For this review, take the finished solid that the model builds, in its own axes (mm). A direction names the side the tool comes from. Coordinates: 2 decimals unless noted, no trailing zeros. Loops run counter-clockwise (first coordinate to the right, second up) from the corner with the lowest first, then second, coordinate; pieces in that order, holes last. Notation, with made-up numbers: (69.5, -15.5) -> (127.5, -15.5) arc R17 cw to (127.5, -8.5) -> close; hole circle Ø8 at (-0.75, 14). An arc over 180 degrees is marked (long way). One line per item, written item: value.
from build123d import *

# Parameters (mm, degrees)
F1_DEPTH = 40
F2_W     = 65
F2_H     = 40
F3_DEPTH = 5
F5_DEPTH = 6


with BuildPart() as f1:
    # F0 (on Top) → F1 (new body)
    with BuildSketch(Plane.XY):
        with BuildLine():
            Line((-3, 43), (1.2426406871, 43))
            ThreePointArc((1.2426406871, 43), (-6, 46), (-3, 38.7573593129))
            Line((-3, 38.7573593129), (-3, 43))
        make_face()
        with BuildLine():
            ThreePointArc((-3, 38.7573593129), (-1.3764116996, 39.0803111054), (0, 40))
            ThreePointArc((0, 40), (0.9196888946, 41.3764116996), (1.2426406871, 43))
            Line((1.2426406871, 43), (-3, 43))
            Line((-3, 43), (-3, 38.7573593129))
        make_face()
        with BuildLine():
            ThreePointArc((-3, 1.2426406871), (-1.3764116996, 0.9196888946), (0, 0))
            Line((0, 0), (0, 40))
            ThreePointArc((0, 40), (-1.3764116996, 39.0803111054), (-3, 38.7573593129))
            Line((-3, 38.7573593129), (-3, 1.2426406871))
        make_face()
        with BuildLine():
            ThreePointArc((1.2426406871, 43), (0.9196888946, 41.3764116996), (0, 40))
            Line((0, 40), (65, 40))
            ThreePointArc((65, 40), (64.0803111054, 41.3764116996), (63.7573593129, 43))
            Line((63.7573593129, 43), (1.2426406871, 43))
        make_face()
        with BuildLine():
            ThreePointArc((72.2426406871, 43), (68, 47.2426406871), (63.7573593129, 43))
            Line((63.7573593129, 43), (68, 43))
            Line((68, 43), (68, 38.7573593129))
            ThreePointArc((68, 38.7573593129), (71, 40), (72.2426406871, 43))
        make_face()
        with BuildLine():
            ThreePointArc((63.7573593129, 43), (64.0803111054, 41.3764116996), (65, 40))
            ThreePointArc((65, 40), (66.3764116996, 39.0803111054), (68, 38.7573593129))
            Line((68, 38.7573593129), (68, 43))
            Line((68, 43), (63.7573593129, 43))
        make_face()
        with BuildLine():
            ThreePointArc((72.2426406871, -3), (71, 0), (68, 1.2426406871))
            Line((68, 1.2426406871), (68, -3))
            Line((68, -3), (63.7573593129, -3))
            ThreePointArc((63.7573593129, -3), (68, -7.2426406871), (72.2426406871, -3))
        make_face()
        with BuildLine():
            ThreePointArc((68, 1.2426406871), (66.3764116996, 0.9196888946), (65, 0))
            ThreePointArc((65, 0), (64.0803111054, -1.3764116996), (63.7573593129, -3))
            Line((63.7573593129, -3), (68, -3))
            Line((68, -3), (68, 1.2426406871))
        make_face()
        with BuildLine():
            ThreePointArc((-3, 1.2426406871), (-6, -6), (1.2426406871, -3))
            Line((1.2426406871, -3), (-3, -3))
            Line((-3, -3), (-3, 1.2426406871))
        make_face()
        with BuildLine():
            ThreePointArc((1.2426406871, -3), (0.9196888946, -1.3764116996), (0, 0))
            ThreePointArc((0, 0), (-1.3764116996, 0.9196888946), (-3, 1.2426406871))
            Line((-3, 1.2426406871), (-3, -3))
            Line((-3, -3), (1.2426406871, -3))
        make_face()
        with BuildLine():
            Line((65, 0), (0, 0))
            ThreePointArc((0, 0), (0.9196888946, -1.3764116996), (1.2426406871, -3))
            Line((1.2426406871, -3), (63.7573593129, -3))
            ThreePointArc((63.7573593129, -3), (64.0803111054, -1.3764116996), (65, 0))
        make_face()
        with BuildLine():
            Line((65, 40), (65, 0))
            ThreePointArc((65, 0), (66.3764116996, 0.9196888946), (68, 1.2426406871))
            Line((68, 1.2426406871), (68, 38.7573593129))
            ThreePointArc((68, 38.7573593129), (66.3764116996, 39.0803111054), (65, 40))
        make_face()
    extrude(amount=F1_DEPTH)

    # F2 (on face) → F3 (join)
    with BuildSketch(Plane(origin=(0, 0, 0), x_dir=(1, 0, 0), z_dir=(0, 0, -1))):
        with BuildLine():
            Line((-3, -1.2426406871), (-3, -38.7573593129))
            ThreePointArc((-3, -38.7573593129), (-6, -46), (1.2426406871, -43))
            Line((1.2426406871, -43), (63.7573593129, -43))
            ThreePointArc((63.7573593129, -43), (71, -46), (68, -38.7573593129))
            Line((68, -38.7573593129), (68, -1.2426406871))
            ThreePointArc((68, -1.2426406871), (71, 6), (63.7573593129, 3))
            Line((63.7573593129, 3), (1.2426406871, 3))
            ThreePointArc((1.2426406871, 3), (-6, 6), (-3, -1.2426406871))
        make_face()
        with Locations((32.5, -20)):
            Rectangle(F2_W, F2_H, mode=Mode.SUBTRACT)
        with Locations((32.5, -20)):
            Rectangle(F2_W, F2_H)
    extrude(amount=F3_DEPTH)

    # F4 (on face) → F5 (join)
    with BuildSketch(Plane.XY):
        with BuildLine():
            ThreePointArc((22, 35), (16.8786796564, 37.1213203436), (19, 32))
            Line((19, 32), (19, 33.65))
            ThreePointArc((19, 33.65), (18.0454058454, 35.9545941546), (20.35, 35))
            Line((20.35, 35), (22, 35))
        make_face()
        with BuildLine():
            Line((19, 33.65), (19, 32))
            ThreePointArc((19, 32), (21.1213203436, 32.8786796564), (22, 35))
            Line((22, 35), (20.35, 35))
            ThreePointArc((20.35, 35), (19.9545941546, 34.0454058454), (19, 33.65))
        make_face()
        with BuildLine():
            Line((46, 33.65), (46, 32))
            ThreePointArc((46, 32), (48.1213203436, 32.8786796564), (49, 35))
            ThreePointArc((49, 35), (46, 38), (43, 35))
            Line((43, 35), (44.65, 35))
            ThreePointArc((44.65, 35), (46, 36.35), (47.35, 35))
            ThreePointArc((47.35, 35), (46.9545941546, 34.0454058454), (46, 33.65))
        make_face()
        with BuildLine():
            ThreePointArc((43, 35), (43.8786796564, 32.8786796564), (46, 32))
            Line((46, 32), (46, 33.65))
            ThreePointArc((46, 33.65), (45.0454058454, 34.0454058454), (44.65, 35))
            Line((44.65, 35), (43, 35))
        make_face()
        with BuildLine():
            ThreePointArc((19, 6.35), (19.9545941546, 5.9545941546), (20.35, 5))
            Line((20.35, 5), (22, 5))
            ThreePointArc((22, 5), (21.1213203436, 7.1213203436), (19, 8))
            Line((19, 8), (19, 6.35))
        make_face()
        with BuildLine():
            Line((22, 5), (20.35, 5))
            ThreePointArc((20.35, 5), (18.0454058454, 4.0454058454), (19, 6.35))
            Line((19, 6.35), (19, 8))
            ThreePointArc((19, 8), (16.8786796564, 2.8786796564), (22, 5))
        make_face()
        with BuildLine():
            ThreePointArc((46, 8), (43.8786796564, 7.1213203436), (43, 5))
            Line((43, 5), (44.65, 5))
            ThreePointArc((44.65, 5), (45.0454058454, 5.9545941546), (46, 6.35))
            Line((46, 6.35), (46, 8))
        make_face()
        with BuildLine():
            Line((44.65, 5), (43, 5))
            ThreePointArc((43, 5), (46, 2), (49, 5))
            ThreePointArc((49, 5), (48.1213203436, 7.1213203436), (46, 8))
            Line((46, 8), (46, 6.35))
            ThreePointArc((46, 6.35), (46.9545941546, 5.9545941546), (47.35, 5))
            ThreePointArc((47.35, 5), (46, 3.65), (44.65, 5))
        make_face()
    extrude(amount=F5_DEPTH)


solid = f1.part
1. Insertion check: pin 1 Ø1 at (y, z) = (10.5, 15.5) entering from +X; pin 2 Ø5 at (x, y) = (46.5, 34.5) entering from +Z; pin 3 Ø2 at (x, z) = (35.5, 10) entering from -Y. Each pin has a flat end and moves straight along its axis. Give the tip position at first contact, or say it passes through.
Return value:
pin 1: stops at x = 68
pin 2: stops at z = 6
pin 3: stops at y = -3
2. The part is to be moulded in two halves that separate along X. For faces 1 (the flat face through (19, 35, 0)), 2 (the flat face through (-3, 20, 18)), 3 (the flat face through (32, 20, -5)), say which applies: pulls with the +X half, pulls with the -X half, needs draft (parallel to the pull), parting line crosses it, or undercut.
Return value:
face 1: undercut
face 2: pulls with the -X half
face 3: needs draft
3. Take a section at A-A, the plane z = 24.5. Give the boundary of the cut face in (x, y).
Return value:
outline: (-3, 1.24) arc R4.24 ccw (long way) to (1.24, -3) -> (63.76, -3) arc R4.24 ccw (long way) to (68, 1.24) -> (68, 38.76) arc R4.24 ccw (long way) to (63.76, 43) -> (1.24, 43) arc R4.24 ccw (long way) to (-3, 38.76) -> close; hole (0, 0) -> (65, 0) -> (65, 40) -> (0, 40) -> close
4. Take a section at C-C, the plane x = 36. Give the boundary of the cut face in (y, z).
Return value:
outline: (-3, -5) -> (43, -5) -> (43, 40) -> (40, 40) -> (40, 0) -> (0, 0) -> (0, 40) -> (-3, 40) -> close
5. For faces 4 (the flat face through (33, 0, 20)), 5 (the flat face through (38.2, 40.3, 40)), list the 3-axis set-ups (+Z, -Z, +X, -X, +Y, -Y) from which the entire face can be reached by the end or side of a thin tool; tool diameter is ignored.
Return value:
face 4: +Z
face 5: +Z, +X, -X, +Y, -Y
6. Take a section at B-B, the plane y = 26.5. Give the boundary of the cut face in (x, z).
Return value:
outline: (-3, -5) -> (68, -5) -> (68, 40) -> (65, 40) -> (65, 0) -> (0, 0) -> (0, 40) -> (-3, 40) -> close
7. To check wall thickness, follow probe 1 along Y at (x, z) = (19, 2.85); probe 2 along X at (y, z) = (35, 1); probe 3 along X at (y, z) = (14, 21). State the ranges of each line that lie inside material, in increasing order. Write a range as from..to.
Return value:
probe 1: y = -3..0, 2..3.65, 6.35..8, 32..33.65, 36.35..38, 40..43
probe 2: x = -3..0, 16..17.65, 20.35..22, 43..44.65, 47.35..49, 65..68
probe 3: x = -3..0, 65..68
